The drawing under review shows one solid part. Ordinate dimensions are in mm from its lowest x, y, z. A direction names the side the tool comes from. Coordinates: 2 decimals unless noted, no trailing zeros. Loops run counter-clockwise (first coordinate to the right, second up) from the corner with the lowest first, then second, coordinate; pieces in that order, holes last. Notation, with made-up numbers: M 51,11.5 L 101,11.5 A8 ccw 101,20.5 Z; hole C 80.5,25.25 d5. An arc over 180 degrees is marked long. Put each result on its own line as item: value.
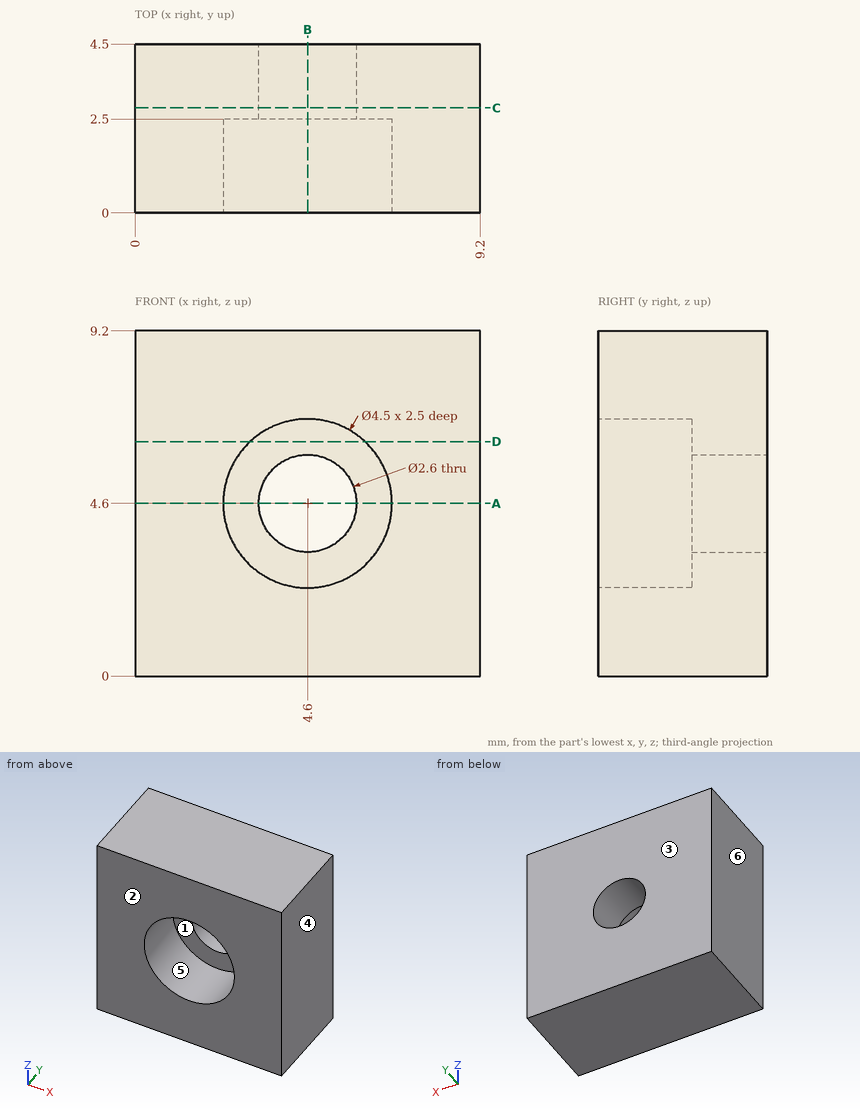
(1) Add section C-C (y = 2.8). Write out the cut boundary in (x, z).
Determined:
outline: M 0,0 L 9.2,0 L 9.2,9.2 L 0,9.2 Z; hole C 4.6,4.6 d2.6
(2) Tool access review of the marked faces 1 and 2: name each direction out of +Z, -Z, +X, -X, +Y, -Y from which nothing blocks a thin tool from reaching the whole face with its end or side.
Determined:
face 1: -Y
face 2: +Z, -Z, +X, -X, -Y
(3) Draft analysis for pull direction X (two halves, no side actions). For the marked faces 3, 4, 5 and 6, state which applies: +X half, -X half, draft (parallel to the pull), parting line (faces both ways), or undercut.
Determined:
face 3: draft
face 4: +X half
face 5: undercut
face 6: -X half
(4) Add section A-A (z = 4.6). Write out the cut boundary in (x, y), plus the area to 4 significant figures.
Determined:
outline: M 0,0 L 2.35,0 L 2.35,2.5 L 3.3,2.5 L 3.3,4.5 L 0,4.5 Z; M 5.9,2.5 L 6.85,2.5 L 6.85,0 L 9.2,0 L 9.2,4.5 L 5.9,4.5 Z
area: 24.95 mm^2
(5) Add section D-D (z = 6.25). Write out the cut boundary in (x, y), plus the area to 3 significant figures.
Determined:
outline: M 0,0 L 3.07,0 L 3.07,2.5 L 6.13,2.5 L 6.13,0 L 9.2,0 L 9.2,4.5 L 0,4.5 Z
area: 33.8 mm^2
(6) Wall thickness on line 1 along Z through (x, y) = (4.6, 0.95); line 2 along Z through (x, y) = (4.6, 3.2): over which ranges is each line inside the solid? List them lowest first. Write a range as [from, to].
Determined:
line 1: z = [0, 2.35], [6.85, 9.2]
line 2: z = [0, 3.3], [5.9, 9.2]
(7) Add section B-B (x = 4.6). Write out the cut boundary in (y, z), plus the area to 4 significant figures.
Determined:
outline: M 0,0 L 4.5,0 L 4.5,3.3 L 2.5,3.3 L 2.5,2.35 L 0,2.35 Z; M 0,6.85 L 2.5,6.85 L 2.5,5.9 L 4.5,5.9 L 4.5,9.2 L 0,9.2 Z
area: 24.95 mm^2
